from build123d import *

# Parameters (mm, degrees)
F1_DEPTH = 20
F3_DEPTH = 25
F4_W     = 34.93
F4_H     = 20
F5_DEPTH = 20
F7_R     = 6.5


with BuildPart() as f1:
    # F0 (on Front) → F1 (new body)
    with BuildSketch(Plane.XZ):
        with BuildLine():
            Line((-10, 348.62), (-10, 501.02))
            Line((-10, 501.02), (-152.88, 501.02))
            Line((-152.88, 501.02), (-76.2948495065, 290.6040283536))
            add(Edge.make_bspline(
                [(-168.28, 0), (-169.5612237815, 52.4820648973), (-175.1232380622, 123.1405186652), (-124.7166168032, 262.8128105239), (-76.2948495065, 290.6040283536)],
                knots=[0, 0, 0, 0, 0.4616253265, 1, 1, 1, 1], degree=3))
            Line((-168.28, 0), (-117.48, 0))
            add(Edge.make_bspline(
                [(-117.48, 0), (-113.0349605269, 49.0087788879), (-103.2300113011, 130.3097354433), (-35.7976257801, 180.8740645647), (0, 174.31)],
                knots=[0, 0, 0, 0, 0.5366116544, 1, 1, 1, 1], degree=3))
            Line((0, 174.31), (0, 348.62))
            Line((0, 348.62), (-10, 348.62))
        make_face()
    extrude(amount=F1_DEPTH)

    # F2 (on face) → F3 (cut)
    with BuildSketch(Plane.XZ):
        Polygon((-38.58, 279.8141206615), (-38.58, 469.27), (-107.5363007859, 469.27), align=None)
    extrude(amount=F3_DEPTH, mode=Mode.SUBTRACT)

    # F4 (on face) → F5 (join)
    with BuildSketch(Plane.XY.offset(501.02)):
        with Locations((-135.415, -10)):
            Rectangle(F4_W, F4_H)
    extrude(amount=F5_DEPTH)

    # F6: F1 across plane


with BuildPart() as f1_1:
    add(f1.part)
    add(f1.part.mirror(Plane.YZ))

    # F7
    f7_edges = [f1_1.edges().sort_by_distance(p)[0] for p in [
        (-107.536301, -10, 469.27),
        (-38.58, -10, 469.27),
        (-38.58, -10, 279.814121),
        (38.58, -10, 279.814121),
        (38.58, -10, 469.27),
        (107.536301, -10, 469.27),
    ]]
    fillet(f7_edges, radius=F7_R)


solid = f1_1.part
Could you check a few things on this model? Use its own coordinates, in mm. A direction names the side the tool comes from. Give positions to 0.01 mm unless a question says otherwise; leave off trailing zeros. Answer as a JSON object with one key per item and string values.
Q1. Suppose I cut it at A-A, the plane y = -13.5. State how many separate pieces and enclosed holes the cut face has, plus the area to 3 significant figures.
Values found:
{"separate pieces": "1", "enclosed holes": "2", "area": "87,300 mm²"}
Q2. For P1, Ø1.5, axis at x = -40.5, z = 441.5, coming from the -Y side; P2, Ø6, axis at y = -8, z = 402.5, coming from the -X side; P3, Ø10, axis at y = -9, z = 431, coming from the +X side; P4, Ø10, axis at y = -5.5, z = 508, coming from the -X side, each with a flat end and sliding along its axis, tell me the tip position at first contact or that it passes through.
Values found:
{"P1": "passes through", "P2": "stops at x = -118.11", "P3": "stops at x = 129.21", "P4": "stops at x = -152.88"}
Q3. If I drill on probe 1 along X at (y, z) = (-2.75, 363.5); probe 2 along X at (y, z) = (-14.25, 411); probe 3 along X at (y, z) = (-5, 334.5), over which ranges is the centre line in solid material (lowest first)? Write a range as [from, to].
Values found:
{"probe 1": "x = [-102.83, -69.04], [-38.58, -10], [10, 38.58], [69.04, 102.83]", "probe 2": "x = [-120.12, -86.33], [-38.58, -10], [10, 38.58], [86.33, 120.12]", "probe 3": "x = [-92.27, -58.48], [-38.58, 38.58], [58.48, 92.27]"}
Q4. For faces 4 (the flat face through (-152.88, -10, 511)), 5 (the cylindrical face through (43.83, -10.14, 310.3)), 6 (the flat face through (63, -10, 501.02)), which set-ups out of +Z, -Z, +X, -X, +Y, -Y let a thin tool reach every point of the face, with its end or its side?
Values found:
{"face 4": "+Z, -X, +Y, -Y", "face 5": "+Y, -Y", "face 6": "+Z, +Y, -Y"}
Q5. If we mould it in two halves opening along X, with no side actions, what happens to faces 1 (the flat face through (136, -10, 521.02)), 2 (the flat face through (115.12, -9.86, 397.28)), 3 (the flat face through (71, -10, 469.27))? For each: pulls with the +X half, pulls with the -X half, needs draft (parallel to the pull), parting line crosses it, or undercut.
Values found:
{"face 1": "needs draft", "face 2": "pulls with the +X half", "face 3": "undercut"}
